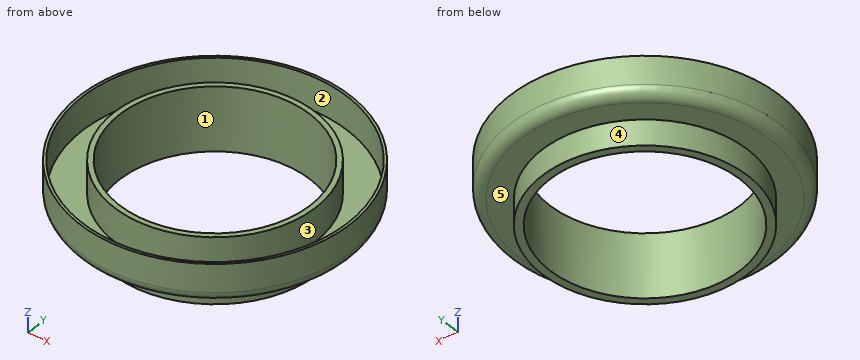
```python
from build123d import *

# Parameters (mm, degrees)
SKETCH055_R        = 52.65
SKETCH055_R_2      = 37.15
PAD023_DEPTH       = 25
SKETCH056_R        = 52.65
SKETCH056_R_2      = 40.15
POCKET003021_DEPTH = 10
SKETCH057_R        = 51.65
SKETCH057_R_2      = 39.15
POCKET003022_DEPTH = 13
FILLET_R           = 4


with BuildPart() as part:
    # Sketch055 → Pad023 (new body)
    with BuildSketch(Plane.XY.offset(80)):
        Circle(SKETCH055_R)
        Circle(SKETCH055_R_2, mode=Mode.SUBTRACT)
    extrude(amount=PAD023_DEPTH)

    # Sketch056 → Pocket003021 (cut)
    with BuildSketch(Plane.XY.offset(80)):
        Circle(SKETCH056_R)
        Circle(SKETCH056_R_2, mode=Mode.SUBTRACT)
    extrude(amount=POCKET003021_DEPTH, mode=Mode.SUBTRACT)

    # Sketch057 → Pocket003022 (cut)
    with BuildSketch(Plane.XY.offset(105)):
        Circle(SKETCH057_R)
        Circle(SKETCH057_R_2, mode=Mode.SUBTRACT)
    extrude(amount=-POCKET003022_DEPTH, mode=Mode.SUBTRACT)

    # Fillet
    fillet_edges = [part.edges().sort_by_distance(p)[0] for p in [
        (-52.65, 0, 90),
    ]]
    fillet(fillet_edges, radius=FILLET_R)


with BuildPart() as part_1:
    # Body010 placement: moved
    add(part.part.moved(Location((0, 0, 14))))


solid = part_1.part
```
Work out the finished part from the listing and answer in its coordinate system (mm). Face numbers are marked on the shaded views. A direction names the side the tool comes from. Give positions to 0.01 mm unless a question says otherwise; leave off trailing zeros. Loops run counter-clockwise (first coordinate to the right, second up) from the corner with the lowest first, then second, coordinate; pieces in that order, holes last. Notation, with made-up numbers: (0.5, 63) -> (39.5, 63) arc R15 cw to (39.5, 92) -> close; hole circle Ø1 at (-34, 46). An arc over 180 degrees is marked (long way). Put each result on its own line as item: value. Start each with the question number.
Item 1: Which of the six approach directions +Z, -Z, +X, -X, +Y, -Y give full straight-line access (tool end or side, diameter ignored) to the marked faces 1 and 2?
Item 2: The part is cut by section C-C (z = 114.5). Give the vertices of the cut face in (x, y).
Item 3: The mould has two halves that part along Y. Classify the marked faces 3, 4 and 5: released by +Y, released by -Y, zero draft, split by the parting line, or undercut.
Item 4: Find the intervals of material crossed by L1, parallel to Y at x = 0, z = 114.75; L2, parallel to Y at x = 0, z = 103.25; L3, parallel to X at y = -7, z = 106.75, in increasing order. Write a range as [from, to].
Item 5: The part is cut by section A-A (x = 0). Give the vertices of the cut face in (y, z).
Item 6: Each of these flat-tipped pins is pushed along its axis until it touches: P1, Ø8, axis at x = -37.5, y = -29.5, coming from the +Z side; P2, Ø10, axis at x = 32, y = -33, coming from the -Z side; P3, Ø10, axis at x = 14.5, z = 101, coming from the -Y side; P4, Ø4, axis at y = 34, z = 107.5, coming from the -X side. Where does it stop, or does it pass through?
Answers below:
1. face 1: +Z, -Z
1. face 2: +Z
2. outline: circle Ø105.3 at (0, 0); circle Ø78.3 at (0, 0); hole circle Ø103.3 at (0, 0); hole circle Ø74.3 at (0, 0)
3. face 3: undercut
3. face 4: split by the parting line
3. face 5: zero draft
4. L1: [-52.65, -51.65], [-39.15, -37.15], [37.15, 39.15], [51.65, 52.65]
4. L2: [-40.15, -37.15], [37.15, 40.15]
4. L3: [-51.98, -51.17], [-38.52, -36.48], [36.48, 38.52], [51.17, 51.98]
5. outline: (-52.65, 108) arc R4 ccw to (-48.65, 104) -> (-40.15, 104) -> (-40.15, 94) -> (-37.15, 94) -> (-37.15, 119) -> (-39.15, 119) -> (-39.15, 106) -> (-51.65, 106) -> (-51.65, 119) -> (-52.65, 119) -> close; (37.15, 94) -> (40.15, 94) -> (40.15, 104) -> (48.65, 104) arc R4 ccw to (52.65, 108) -> (52.65, 119) -> (51.65, 119) -> (51.65, 106) -> (39.15, 106) -> (39.15, 119) -> (37.15, 119) -> close
6. P1: z = 119
6. P2: z = 104
6. P3: y = -50.32
6. P4: x = -41.79
